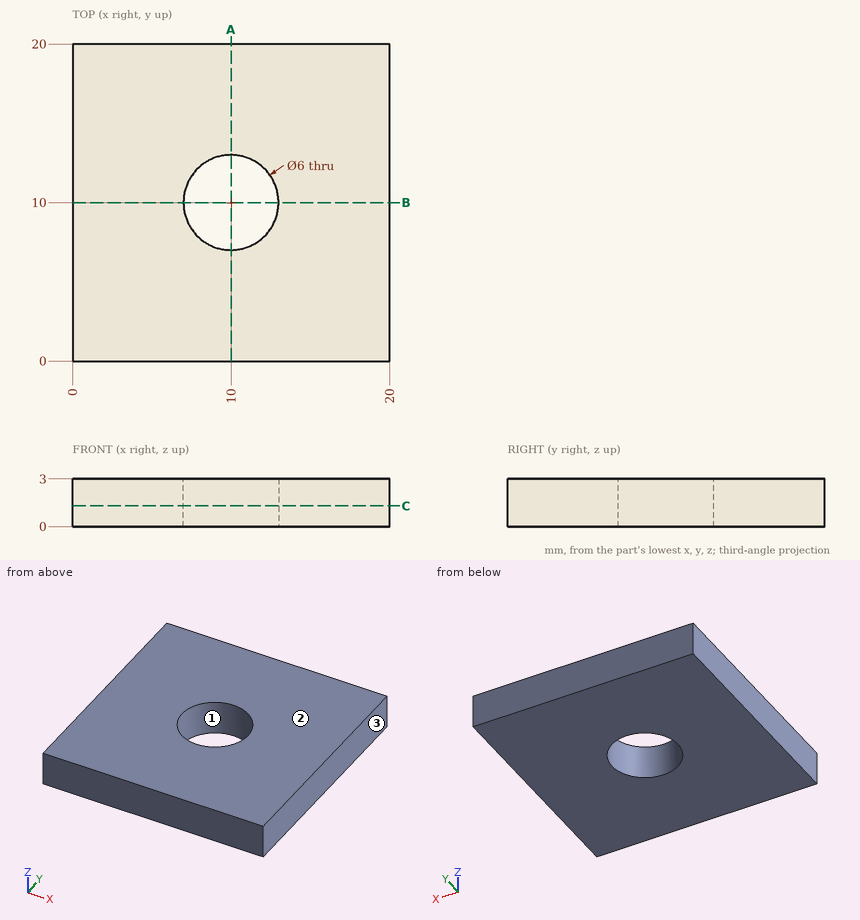
Design review of the part shown in the three views and the two pictorial views. Dimensions are in mm from the part's minimum x, y and z. Round coordinates to 2 decimals unless told otherwise and drop trailing zeros. Write each loop counter-clockwise with the first axis right and the second up, starting at its lowest first coordinate (ties: lowest second). Pieces come first, ordered by that corner, then holes.
Item 1: For probe 1 along Y at (x, z) = (10, 0.9); probe 2 along X at (y, z) = (8, 0.55); probe 3 along X at (y, z) = (11, 1.65), list the stretches that pass through material, from the lowest coordinate up.
Item 2: Clearance check with a flat-ended pin moving along its axis: pin 1 Ø8 at (x, y) = (3, 12) entering from -Z. State where the tip first meets the part, or that it passes through.
Item 3: We need section A-A on x = 10. Write out the cut boundary in (y, z), and give its area (3 significant figures).
Item 4: We need section C-C on z = 1.3. Write out the cut boundary in (x, y), and give its area (3 significant figures).
Item 5: The part is to be moulded in two halves that separate along X. For the marked faces 1, 2 and 3, say which applies: +X half, -X half, draft (parallel to the pull), parting line (faces both ways), or undercut.
Returned:
1. probe 1: y = 0 to 7, 13 to 20
1. probe 2: x = 0 to 7.76, 12.24 to 20
1. probe 3: x = 0 to 7.17, 12.83 to 20
2. pin 1: stops at z = 0
3. outline: (0, 0) - (7, 0) - (7, 3) - (0, 3) - close; (13, 0) - (20, 0) - (20, 3) - (13, 3) - close
3. area: 42.0 mm2
4. outline: (0, 0) - (20, 0) - (20, 20) - (0, 20) - close; hole circle Ø6 at (10, 10)
4. area: 372 mm2
5. face 1: undercut
5. face 2: draft
5. face 3: +X half
